Geometry check sheet. Reference: the model listing, model coordinates, mm. Face numbers are marked on the shaded views. A direction names the side the tool comes from. Give positions to 0.01 mm unless a question says otherwise; leave off trailing zeros. Order: outer loops, then holes, each group sorted by start corner. A loop starts at its lowest first (then second) coordinate and runs counter-clockwise, first axis right, second up. Notation, with made-up numbers: (14, 57) - (45, 57) arc R33 cw to (45, 87) - close; hole circle Ø4 at (-38, 52). An arc over 180 degrees is marked (long way). Put each result on its own line as item: value. Start each with the question number.
```python
from build123d import *

# Parameters (mm, degrees)
SKETCH1_W               = 90
SKETCH1_H               = 110
BOSS_EXTRUDE1_DEPTH     = 2.5
CUT_EXTRUDE1_DEPTH      = 72.107313267
SKETCH6_R               = 1.6
CUT_EXTRUDE4_DEPTH      = 72.107313267
SKETCH3_W               = 90
SKETCH3_H               = 110
SKETCH3_W_2             = 86
SKETCH3_H_2             = 106
BOSS_EXTRUDE2_DEPTH     = 43.5
SKETCH4_W               = 7
SKETCH4_H               = 7
BOSS_EXTRUDE3_DEPTH     = 5
CUT_EXTRUDE3_REACH      = 86.652
SKETCH5_R               = 2.4
MIRROR2_COPY_1_SKETCH_W = 7
MIRROR2_COPY_1_SKETCH_H = 7
MIRROR2_COPY_1_DEPTH    = 5
MIRROR2_COPY_2_REACH    = 86.652
MIRROR2_COPY_2_SKETCH_R = 2.4
SKETCH8_R               = 3
CUT_EXTRUDE5_DEPTH      = 10
CUT_EXTRUDE6_DEPTH      = 116.06954419
CUT_EXTRUDE7_REACH      = 129.44
SKETCH12_R              = 2
CUT_EXTRUDE8_DEPTH      = 5
CHAMFER1_SIZE           = 0.6
CHAMFER1_SIZE_2         = 1.039230485
FILLET1_R               = 3.5


with BuildPart() as part:
    # Sketch1 → Boss-Extrude1 (new body)
    with BuildSketch(Plane(origin=(0, 0, 0), x_dir=(1, 0, 0), z_dir=(0, 1, 0))):
        Rectangle(SKETCH1_W, SKETCH1_H)
    extrude(amount=BOSS_EXTRUDE1_DEPTH)

    # Sketch2 → Cut-Extrude1 (cut, through all)
    with BuildSketch(Plane(origin=(0, 2.5, 0), x_dir=(1, 0, 0), z_dir=(0, 1, 0))):
        with BuildLine():
            Line((-40, 50), (-16.83333333, 50))
            ThreePointArc((-16.83333333, 50), (-13.33333333, 46.5), (-9.83333333, 50))
            Line((-9.83333333, 50), (23.5, 50))
            ThreePointArc((23.5, 50), (27, 46.5), (30.5, 50))
            Line((30.5, 50), (40, 50))
            Line((40, 50), (40, -50))
            Line((40, -50), (25.6874353, -50))
            ThreePointArc((25.6874353, -50), (22.333333333, -47.5), (18.979231367, -50))
            Line((18.979231367, -50), (-14.8125647, -50))
            ThreePointArc((-14.8125647, -50), (-18.166666667, -47.5), (-21.520768633, -50))
            Line((-21.520768633, -50), (-40, -50))
            Line((-40, -50), (-40, 50))
        make_face()
    extrude(amount=-CUT_EXTRUDE1_DEPTH, mode=Mode.SUBTRACT)

    # Sketch6 → Cut-Extrude4 (cut, through all)
    with BuildSketch(Plane(origin=(0, 2.5, 0), x_dir=(1, 0, 0), z_dir=(0, 1, 0))):
        with Locations(Location((-13.33333333, 50, 0), (0, 0, 270))):
            Circle(SKETCH6_R)
        with Locations(Location((27, 50, 0), (0, 0, 270))):
            Circle(SKETCH6_R)
        with Locations(Location((22.333333333, -51, 0), (0, 0, 270))):
            Circle(SKETCH6_R)
        with Locations(Location((-18.166666667, -51, 0), (0, 0, 270))):
            Circle(SKETCH6_R)
    extrude(amount=-CUT_EXTRUDE4_DEPTH, mode=Mode.SUBTRACT)

    # Sketch3 → Boss-Extrude2 (add)
    with BuildSketch(Plane(origin=(0, 2.5, 0), x_dir=(1, 0, 0), z_dir=(0, 1, 0))):
        Rectangle(SKETCH3_W, SKETCH3_H)
        Rectangle(SKETCH3_W_2, SKETCH3_H_2, mode=Mode.SUBTRACT)
    extrude(amount=BOSS_EXTRUDE2_DEPTH)

    # Sketch4 → Boss-Extrude3 (add)
    with BuildSketch(Plane(origin=(0, 46, 0), x_dir=(1, 0, 0), z_dir=(0, 1, 0))):
        with Locations((-39.5, 49.5)):
            Rectangle(SKETCH4_W, SKETCH4_H)
    boss_extrude3 = extrude(amount=-BOSS_EXTRUDE3_DEPTH)

    # Sketch5 → Cut-Extrude3 (cut, up to next)
    with BuildSketch(Plane(origin=(0, 46, 0), x_dir=(1, 0, 0), z_dir=(0, 1, 0)), mode=Mode.PRIVATE) as cut_extrude3_sk1:
        with Locations(Location((-40, 50, 0), (0, 0, 270))):
            Circle(SKETCH5_R)
    cut_extrude3_tool1 = extrude(cut_extrude3_sk1.sketch, amount=-CUT_EXTRUDE3_REACH, mode=Mode.PRIVATE) & part.part
    cut_extrude3 = cut_extrude3_tool1.solids().sort_by_distance((-40, 46, -50))[0]
    add(cut_extrude3, mode=Mode.SUBTRACT)

    # Mirror1: Boss-Extrude3, Cut-Extrude3 across plane
    add(boss_extrude3.mirror(Plane(origin=(0, 0, 0), x_dir=(0, 0, 1), z_dir=(1, 0, 0))))
    add(cut_extrude3.mirror(Plane(origin=(0, 0, 0), x_dir=(0, 0, 1), z_dir=(1, 0, 0))), mode=Mode.SUBTRACT)

    # Mirror2: Boss-Extrude3, Cut-Extrude3 across plane
    add(boss_extrude3.mirror(Plane.XY))
    add(cut_extrude3.mirror(Plane.XY), mode=Mode.SUBTRACT)

    # Mirror2 copy 1 sketch → Mirror2 copy 1 (add)
    with BuildSketch(Plane(origin=(0, 46, 0), x_dir=(-1, 0, 0), z_dir=(0, 1, 0))):
        with Locations((-39.5, 49.5)):
            Rectangle(MIRROR2_COPY_1_SKETCH_W, MIRROR2_COPY_1_SKETCH_H)
    extrude(amount=-MIRROR2_COPY_1_DEPTH)

    # Mirror2 copy 2 sketch → Mirror2 copy 2 (cut, up to next)
    with BuildSketch(Plane(origin=(0, 46, 0), x_dir=(-1, 0, 0), z_dir=(0, 1, 0)), mode=Mode.PRIVATE) as mirror2_copy_2_sk1:
        with Locations(Location((-40, 50, 0), (0, 0, 270))):
            Circle(MIRROR2_COPY_2_SKETCH_R)
    mirror2_copy_2_tool1 = extrude(mirror2_copy_2_sk1.sketch, amount=-MIRROR2_COPY_2_REACH, mode=Mode.PRIVATE) & part.part
    add(mirror2_copy_2_tool1.solids().sort_by_distance((40, 46, 50))[0], mode=Mode.SUBTRACT)

    # Sketch8 → Cut-Extrude5 (cut)
    with BuildSketch(Plane(origin=(0, 2.5, 0), x_dir=(1, 0, 0), z_dir=(0, 1, 0))):
        with Locations((-18.166666667, -51)):
            Circle(SKETCH8_R)
        with Locations((22.333333333, -51)):
            Circle(SKETCH8_R)
    extrude(amount=CUT_EXTRUDE5_DEPTH, mode=Mode.SUBTRACT)

    # Sketch9 → Cut-Extrude6 (cut, through all)
    with BuildSketch(Plane.ZY.offset(45)):
        with BuildLine():
            Line((-44, 6), (-44, 0))
            Line((-44, 0), (-22, 0))
            Line((-22, 0), (-22, 6))
            ThreePointArc((-22, 6), (-33, 9.296706912), (-44, 6))
        make_face()
        with BuildLine():
            Line((29, 0), (43, 0))
            Line((43, 0), (43, 5))
            ThreePointArc((43, 5), (36, 6.143346385), (29, 5))
            Line((29, 5), (29, 0))
        make_face()
    extrude(amount=-CUT_EXTRUDE6_DEPTH, mode=Mode.SUBTRACT)

    # Sketch10 → Cut-Extrude7 (cut, up to next)
    with BuildSketch(Plane(origin=(0, 0, -55), x_dir=(-1, 0, 0), z_dir=(0, 0, -1)), mode=Mode.PRIVATE) as cut_extrude7_sk1:
        with BuildLine():
            Line((14, 46), (30, 46))
            Line((30, 46), (30, 45.8))
            ThreePointArc((30, 45.8), (29.472792206, 44.527207794), (28.2, 44))
            Line((28.2, 44), (15.8, 44))
            ThreePointArc((15.8, 44), (14.527207794, 44.527207794), (14, 45.8))
            Line((14, 45.8), (14, 46))
        make_face()
    cut_extrude7_tool1 = extrude(cut_extrude7_sk1.sketch, amount=-CUT_EXTRUDE7_REACH, mode=Mode.PRIVATE) & part.part
    # Sketch10 → Cut-Extrude7 (cut, up to next)
    with BuildSketch(Plane(origin=(0, 0, -55), x_dir=(-1, 0, 0), z_dir=(0, 0, -1)), mode=Mode.PRIVATE) as cut_extrude7_sk2:
        with BuildLine():
            Line((-30, 46), (-30, 45.8))
            ThreePointArc((-30, 45.8), (-29.472792206, 44.527207794), (-28.2, 44))
            Line((-28.2, 44), (-15.8, 44))
            ThreePointArc((-15.8, 44), (-14.527207794, 44.527207794), (-14, 45.8))
            Line((-14, 45.8), (-14, 46))
            Line((-14, 46), (-30, 46))
        make_face()
    cut_extrude7_tool2 = extrude(cut_extrude7_sk2.sketch, amount=-CUT_EXTRUDE7_REACH, mode=Mode.PRIVATE) & part.part
    add(cut_extrude7_tool1.solids().sort_by_distance((-22, 45.027165, -55))[0], mode=Mode.SUBTRACT)
    add(cut_extrude7_tool2.solids().sort_by_distance((22, 45.027165, -55))[0], mode=Mode.SUBTRACT)

    # Sketch12 → Cut-Extrude8 (cut)
    with BuildSketch(Plane(origin=(0, 0, 0), x_dir=(1, 0, 0), z_dir=(0, 1, 0))):
        with Locations((-40, -50)):
            Circle(SKETCH12_R)
        with Locations((40, -50)):
            Circle(SKETCH12_R)
        with Locations((-40, 50)):
            Circle(SKETCH12_R)
        with Locations((40, 50)):
            Circle(SKETCH12_R)
    extrude(amount=CUT_EXTRUDE8_DEPTH, mode=Mode.SUBTRACT)

    # Chamfer1
    # the kernel refuses this chamfer: 1.039230485, 0.6 mm, written as the material it takes off along each edge
    with BuildSketch(Plane(origin=(-40, 41, -50), x_dir=(0, 0, 1), z_dir=(-1, 0, 0))) as chamfer1_piece_1_section:
        Polygon((2.4 + CHAMFER1_SIZE, 0), (2.4, CHAMFER1_SIZE_2), (2.4, 0), align=None)
    chamfer1_piece_1 = revolve(axis=Axis((-40, 41, -50), (0, 1, 0)), mode=Mode.PRIVATE)
    chamfer1_piece_1 = split(chamfer1_piece_1, bisect_by=Plane(origin=(-43, 41.510650162, -52.684472026), z_dir=(1, 0, 0)), keep=Keep.TOP, mode=Mode.PRIVATE)
    chamfer1_piece_1 = split(chamfer1_piece_1, bisect_by=Plane(origin=(-40, 41.510650162, -53), z_dir=(0, 0, 1)), keep=Keep.TOP, mode=Mode.PRIVATE)
    add(chamfer1_piece_1, mode=Mode.SUBTRACT)
    with BuildSketch(Plane(origin=(40, 41, -50), x_dir=(0, 0, 1), z_dir=(1, 0, 0))) as chamfer1_piece_2_section:
        Polygon((2.4 + CHAMFER1_SIZE_2, 0), (2.4, -CHAMFER1_SIZE), (2.4, 0), align=None)
    chamfer1_piece_2 = revolve(axis=Axis((40, 41, -50), (0, -1, 0)), mode=Mode.PRIVATE)
    chamfer1_piece_2 = split(chamfer1_piece_2, bisect_by=Plane(origin=(40, 41.284402775, -53), z_dir=(0, 0, 1)), keep=Keep.TOP, mode=Mode.PRIVATE)
    chamfer1_piece_2 = split(chamfer1_piece_2, bisect_by=Plane(origin=(43, 41.284402775, -52.91061018), z_dir=(-1, 0, 0)), keep=Keep.TOP, mode=Mode.PRIVATE)
    add(chamfer1_piece_2, mode=Mode.SUBTRACT)
    with BuildSketch(Plane(origin=(40, 41, 50), x_dir=(0, 0, -1), z_dir=(1, 0, 0))) as chamfer1_piece_3_section:
        Polygon((2.4 + CHAMFER1_SIZE, 0), (2.4, CHAMFER1_SIZE_2), (2.4, 0), align=None)
    chamfer1_piece_3 = revolve(axis=Axis((40, 41, 50), (0, 1, 0)), mode=Mode.PRIVATE)
    chamfer1_piece_3 = split(chamfer1_piece_3, bisect_by=Plane(origin=(43, 41.510650162, 52.684472026), z_dir=(-1, 0, 0)), keep=Keep.TOP, mode=Mode.PRIVATE)
    chamfer1_piece_3 = split(chamfer1_piece_3, bisect_by=Plane(origin=(40, 41.510650162, 53), z_dir=(0, 0, -1)), keep=Keep.TOP, mode=Mode.PRIVATE)
    add(chamfer1_piece_3, mode=Mode.SUBTRACT)
    with BuildSketch(Plane(origin=(-40, 41, 50), x_dir=(0, 0, -1), z_dir=(-1, 0, 0))) as chamfer1_piece_4_section:
        Polygon((2.4 + CHAMFER1_SIZE_2, 0), (2.4, -CHAMFER1_SIZE), (2.4, 0), align=None)
    chamfer1_piece_4 = revolve(axis=Axis((-40, 41, 50), (0, -1, 0)), mode=Mode.PRIVATE)
    chamfer1_piece_4 = split(chamfer1_piece_4, bisect_by=Plane(origin=(-43, 41.284402775, 52.91061018), z_dir=(1, 0, 0)), keep=Keep.TOP, mode=Mode.PRIVATE)
    chamfer1_piece_4 = split(chamfer1_piece_4, bisect_by=Plane(origin=(-40, 41.284402775, 53), z_dir=(0, 0, -1)), keep=Keep.TOP, mode=Mode.PRIVATE)
    add(chamfer1_piece_4, mode=Mode.SUBTRACT)

    # Fillet1
    fillet1_edges = [part.edges().sort_by_distance(p)[0] for p in [
        (36, 43.5, -46),
        (36, 43.5, 46),
        (-36, 43.5, 46),
        (-36, 43.5, -46),
    ]]
    fillet(fillet1_edges, radius=FILLET1_R)


solid = part.part
```
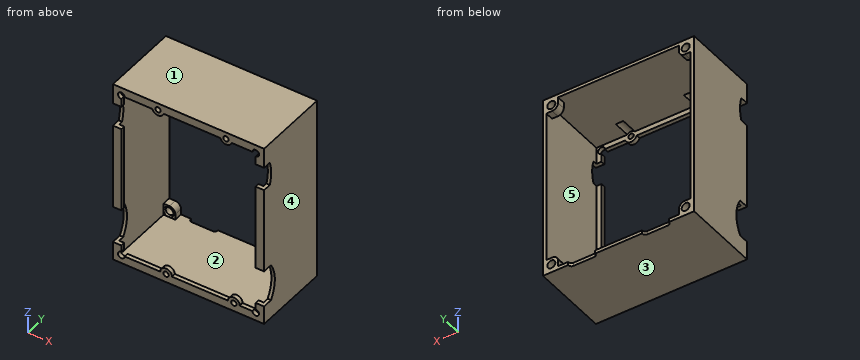
Item 1: Gauge pin test, flat ends, axial feed: pin 1 Ø3 at (x, z) = (27, -50) entering from +Y; pin 2 Ø4.5 at (x, z) = (-40, -50) entering from +Y. Record the tip position at first contact, or that the pin passes through.
Item 2: Thickness scan on line 1 along X through (y, z) = (44.95, -50); line 2 along X through (y, z) = (10.5, 36.5); line 3 along Z through (x, y) = (-21, 28). Record the ranges inside material, lowest first.
Item 3: Set-up check for the marked faces 1 and 2: record each of +Z, -Z, +X, -X, +Y, -Y from which the full face is reachable in a straight line by a thin tool's end or side.
Item 4: Release check for a two-part mould opening along Z. For the marked faces 3, 4 and 5 record: +Z half, -Z half, draft (parallel to the pull), parting line (faces both ways), or undercut.
Item 5: Cross-section at A-A (z = -14). Enter the section's corners in (x, y), and give its area (3 significant figures).
Item 6: Cross-section at B-B (x = -23). Enter the section's corners in (y, z), and give its area (3 significant figures).
Item 7: Cross-section at C-C (y = 27). Enter the section's corners in (x, z).
Recorded:
1. pin 1: passes through
1. pin 2: stops at y = 2.5
2. line 1: x = -45 to -42.4, -37.6 to -36, 36 to 37.6, 42.4 to 45
2. line 2: x = -45 to -43, 43 to 45
2. line 3: z = -55 to -53, 53 to 55
3. face 1: +Z, +X, -X, +Y, -Y
3. face 2: none
4. face 3: -Z half
4. face 4: draft
4. face 5: undercut
5. outline: (-45, 0) - (-40, 0) - (-40, 2.5) - (-43, 2.5) - (-43, 46) - (-45, 46) - close; (40, 0) - (45, 0) - (45, 46) - (43, 46) - (43, 2.5) - (40, 2.5) - close
5. area: 199 mm^2
6. outline: (0, -55) - (44, -55) - (44, -53) - (2.5, -53) - (2.5, -50) - (0, -50) - close; (0, 50) - (2.5, 50) - (2.5, 53) - (46, 53) - (46, 55) - (0, 55) - close
6. area: 195 mm^2
7. outline: (-45, -55) - (45, -55) - (45, 55) - (-45, 55) - close; hole (-43, -53) - (43, -53) - (43, 53) - (-43, 53) - close
